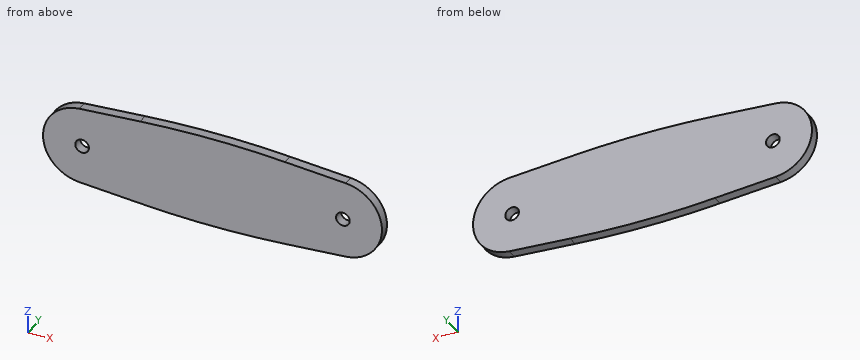
from build123d import *

# Parameters (mm, degrees)
SKETCH_1_R      = 2.1
EXTRUDE_1_DEPTH = 3
FILLET_1_R      = 300


with BuildPart() as part:
    # 草图1 → 凸台-拉伸1 (new body)
    with BuildSketch(Plane(origin=(0, 0, 0), x_dir=(1, 0, 0), z_dir=(0, 1, 0))):
        with BuildLine():
            Line((-0.887671233, 11.967123288), (40, 15))
            Line((40, 15), (80.887671233, 11.967123288))
            ThreePointArc((80.887671233, 11.967123288), (92, 0), (80.887671233, -11.967123288))
            Line((80.887671233, -11.967123288), (40, -15))
            Line((40, -15), (-0.887671233, -11.967123288))
            ThreePointArc((-0.887671233, -11.967123288), (-12, 0), (-0.887671233, 11.967123288))
        make_face()
        with Locations(Location((0, 0, 0), (0, 0, 270))):
            Circle(SKETCH_1_R, mode=Mode.SUBTRACT)
        with Locations(Location((80, 0, 0), (0, 0, 270))):
            Circle(SKETCH_1_R, mode=Mode.SUBTRACT)
    extrude(amount=EXTRUDE_1_DEPTH)

    # 圆角1
    fillet_1_edges = [part.edges().sort_by_distance(p)[0] for p in [
        (40, 1.5, 15),
        (40, 1.5, -15),
    ]]
    fillet(fillet_1_edges, radius=FILLET_1_R)


solid = part.part
Input: part model. Units: mm. Frame: model coordinates. Round coordinates to 2 decimals unless told otherwise and drop trailing zeros. Loops run counter-clockwise (first coordinate to the right, second up) from the corner with the lowest first, then second, coordinate; pieces in that order, holes last. Notation, with made-up numbers: (46, -26) -> (60, -26) arc R25 ccw to (60, 5) -> close; hole circle Ø2 at (0, -8). An arc over 180 degrees is marked (long way). Answer as a JSON object with one key per item and string values. Group by question number.
1) Section query C-C on x = 0. Output: boundary loops of the cut face in (y, z).
2) Section query D-D on x = 72.5. Output: boundary loops of the cut face in (y, z).
3) Section query B-B on y = 1.6. Output: boundary loops of the cut face in (x, z).
4) Ray query, L1, parallel to X at y = 2.3, z = 0.5; L2, parallel to Z at x = 27, y = 1.85; L3, parallel to Z at x = 4.5, y = 2.35. Return the intervals inside material, ascending.
5) Section query A-A on z = 0. Output: boundary loops of the cut face in (x, y), plus the area to 3 significant figures.
6) Pin query (flat end, axial travel): pin 1 (1.5 mm diameter, centred on y = 1.5, z = -11, fed in from -X). Return the tip coordinate at first contact, or that it passes through.
Reply:
{
 "1": {"outline": "(0, -12.03) -> (3, -12.03) -> (3, -2.1) -> (0, -2.1) -> close; (0, 2.1) -> (3, 2.1) -> (3, 12.03) -> (0, 12.03) -> close"},
 "2": {"outline": "(0, -12.59) -> (3, -12.59) -> (3, 12.59) -> (0, 12.59) -> close"},
 "3": {"outline": "(-0.89, -11.97) -> (17.81, -13.35) arc R300 ccw to (62.19, -13.35) -> (80.89, -11.97) arc R12 ccw to (80.89, 11.97) -> (62.19, 13.35) arc R300 ccw to (17.81, 13.35) -> (-0.89, 11.97) arc R12 ccw to start; hole circle Ø4.2 at (0, 0); hole circle Ø4.2 at (80, 0)"},
 "4": {"L1": "x = -11.99 to -2.04, 2.04 to 77.96, 82.04 to 91.99", "L2": "z = -13.89 to 13.89", "L3": "z = -12.37 to 12.37"},
 "5": {"outline": "(-12, 0) -> (-2.1, 0) -> (-2.1, 3) -> (-12, 3) -> close; (2.1, 0) -> (77.9, 0) -> (77.9, 3) -> (2.1, 3) -> close; (82.1, 0) -> (92, 0) -> (92, 3) -> (82.1, 3) -> close", "area": "287 mm2"},
 "6": {"pin 1": "stops at x = -6.24"}
}
